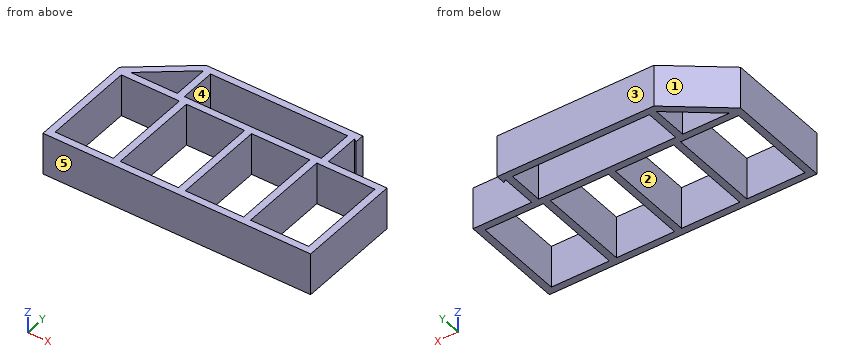
from build123d import *

# Parameters (mm, degrees)
F0_W     = 50.8
F0_H     = 261.669054
F0_H_2   = 660.4
F1_DEPTH = 304.8


with BuildPart() as f1:
    # F0 (on Top) → F1 (new body)
    with BuildSketch(Plane.XY):
        Polygon((564.666493, 625.426641), (564.666493, 693.469054), (-564.666493, 693.469054), (-965.2, 381), (-882.611341, 381), (-547.19501, 642.669054), (-496.39501, 642.669054), (491.437937, 642.669054), (542.237937, 642.669054), align=None)
        with Locations((-521.79501, 511.834527)):
            Rectangle(F0_W, F0_H)
        with Locations((516.837937, 511.834527)):
            Rectangle(F0_W, F0_H)
        Polygon((965.2, -381), (965.2, 381), (882.611341, 381), (542.237937, 381), (491.437937, 381), (-496.39501, 381), (-547.19501, 381), (-882.611341, 381), (-965.2, 381), (-965.2, -381), align=None)
        Polygon((495.3, 330.2), (914.4, 330.2), (914.4, -330.2), (495.3, -330.2), (444.5, -330.2), (25.4, -330.2), (-25.4, -330.2), (-444.5, -330.2), (-495.3, -330.2), (-914.4, -330.2), (-914.4, 330.2), (-495.3, 330.2), (-444.5, 330.2), (-25.4, 330.2), (25.4, 330.2), (444.5, 330.2), align=None, mode=Mode.SUBTRACT)
        with Locations((469.9, 0)):
            Rectangle(F0_W, F0_H_2)
        Rectangle(F0_W, F0_H_2)
        with Locations((-469.9, 0)):
            Rectangle(F0_W, F0_H_2)
    extrude(amount=F1_DEPTH)


solid = f1.part
Geometry check sheet. Reference: the model listing, model coordinates, mm. Face numbers are marked on the shaded views. A direction names the side the tool comes from. Coordinates: 2 decimals unless noted, no trailing zeros. Order: outer loops, then holes, each group sorted by start corner. A loop starts at its lowest first (then second) coordinate and runs counter-clockwise, first axis right, second up. Notation, with made-up numbers: (-35, -24) - (5, -24) arc R11 ccw to (5, -12) - close; hole circle Ø11 at (73, 29). An arc over 180 degrees is marked (long way). Answer in a Markdown table with one row per item. Add a question column.
1) Release check for a two-part mould opening along Y. For the marked faces 3, 4 and 5 record: +Y half, -Y half, draft (parallel to the pull), parting line (faces both ways), or undercut.
2) Cross-section at A-A, the plane x = -115. Record the cut outline in (y, z), then the cut area to 3 significant figures.
3) Set-up check for the marked faces 1 and 2: record each of +Z, -Z, +X, -X, +Y, -Y from which the full face is reachable in a straight line by a thin tool's end or side.
4) Cross-section at C-C, the plane z = 41. State how many separate pieces and enclosed holes the cut face has, then the cut area to 3 significant figures.
5) Cross-section at B-B, the plane y = -58. Record the cut outline in (x, z), then the cut area to 3 significant figures.
6) Cross-section at D-D, the plane x = 652. Record the cut outline in (y, z), then the cut area to 3 significant figures.
7) Gauge pin test, flat ends, axial feed: P1, Ø20.5, axis at y = 644, z = 156, coming from the +X side; P2, Ø5, axis at y = 418, z = 170.5, coming from the -X side. Record the tip position at first contact, or that the pin passes through.
8) Material ranges on line 1 along Y through (x, z) = (-179, 159); line 2 along X through (y, z) = (330, 27); line 3 along Y through (x, z) = (619, 66.5), recorded low to high. Write a range as [from, to].
Check result:
| question | item | result |
|---|---|---|
| 1 | face 3 | +Y half |
| 1 | face 4 | undercut |
| 1 | face 5 | -Y half |
| 2 | outline | (-381, 0) - (-330.2, 0) - (-330.2, 304.8) - (-381, 304.8) - close; (330.2, 0) - (381, 0) - (381, 304.8) - (330.2, 304.8) - close; (642.67, 0) - (693.47, 0) - (693.47, 304.8) - (642.67, 304.8) - close |
| 2 | area | 46,500 mm² |
| 3 | face 1 | +Z, -Z, -X, +Y |
| 3 | face 2 | +Z, -Z |
| 4 | separate pieces | 1 |
| 4 | enclosed holes | 6 |
| 4 | area | 471,000 mm² |
| 5 | outline | (-965.2, 0) - (-914.4, 0) - (-914.4, 304.8) - (-965.2, 304.8) - close; (-495.3, 0) - (-444.5, 0) - (-444.5, 304.8) - (-495.3, 304.8) - close; (-25.4, 0) - (25.4, 0) - (25.4, 304.8) - (-25.4, 304.8) - close; (444.5, 0) - (495.3, 0) - (495.3, 304.8) - (444.5, 304.8) - close; (914.4, 0) - (965.2, 0) - (965.2, 304.8) - (914.4, 304.8) - close |
| 5 | area | 77,400 mm² |
| 6 | outline | (-381, 0) - (-330.2, 0) - (-330.2, 304.8) - (-381, 304.8) - close; (330.2, 0) - (381, 0) - (381, 304.8) - (330.2, 304.8) - close |
| 6 | area | 31,000 mm² |
| 7 | P1 | stops at x = 564.67 |
| 7 | P2 | stops at x = -920.98 |
| 8 | line 1 | y = [-381, -330.2], [330.2, 381], [642.67, 693.47] |
| 8 | line 2 | x = [-965.2, -914.4], [-495.3, -444.5], [-25.4, 25.4], [444.5, 495.3], [914.4, 965.2] |
| 8 | line 3 | y = [-381, -330.2], [330.2, 381] |
